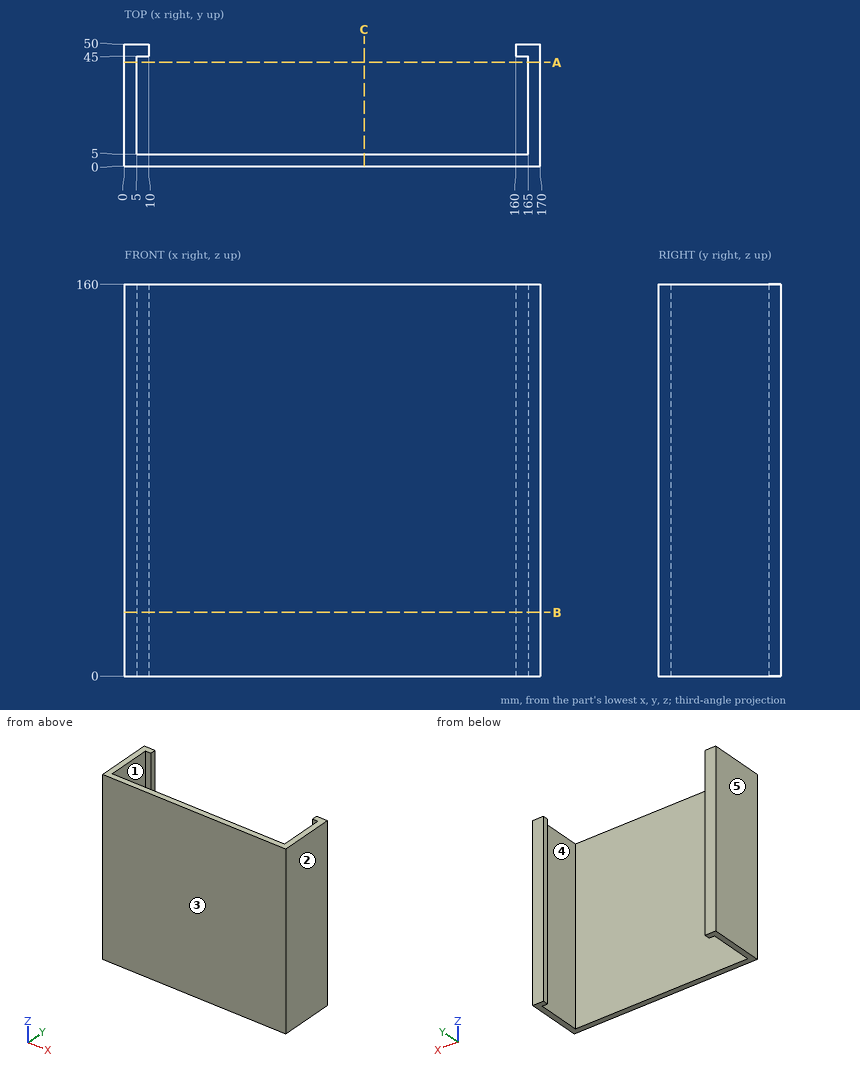
Geometry check sheet. Reference: drawing and pictorial views, mm from the part's lowest x, y, z. A direction names the side the tool comes from. Round coordinates to 2 decimals unless told otherwise and drop trailing zeros. Loops run counter-clockwise (first coordinate to the right, second up) from the corner with the lowest first, then second, coordinate; pieces in that order, holes last.
1. Scan lines: probe 1 along X at (y, z) = (47, 111.5); probe 2 along X at (y, z) = (38, 44.5); probe 3 along Y at (x, z) = (54, 127). Record each from-to range of solid material in increasing order.
2. Gauge pin test, flat end, axial feed: pin 1 Ø1.5 at (x, z) = (35, 46.5) entering from +Y. Record the tip position at first contact, or that the pin passes through.
3. Sectioned sample at A-A on y = 42.5. Record the boundary of the cut face in (x, z).
4. Sectioned sample at C-C on x = 98. Record the boundary of the cut face in (y, z).
5. Set-up check for the marked faces 4 and 5: record each of +Z, -Z, +X, -X, +Y, -Y from which the full face is reachable in a straight line by a thin tool's end or side.
6. Sectioned sample at B-B on z = 26. Record the boundary of the cut face in (x, y).
7. Mould release check, pull along Y, two halves, no side actions. Record for the marked faces 1, 2 and 3: released by +Y, released by -Y, zero draft, split by the parting line, or undercut.
Recorded:
1. probe 1: x = 0 to 10, 160 to 170
1. probe 2: x = 0 to 5, 165 to 170
1. probe 3: y = 0 to 5
2. pin 1: stops at y = 5
3. outline: (0, 0) - (5, 0) - (5, 160) - (0, 160) - close; (165, 0) - (170, 0) - (170, 160) - (165, 160) - close
4. outline: (0, 0) - (5, 0) - (5, 160) - (0, 160) - close
5. face 4: +Z, -Z
5. face 5: +Z, -Z, -X, +Y, -Y
6. outline: (0, 0) - (170, 0) - (170, 50) - (160, 50) - (160, 45) - (165, 45) - (165, 5) - (5, 5) - (5, 45) - (10, 45) - (10, 50) - (0, 50) - close
7. face 1: undercut
7. face 2: zero draft
7. face 3: released by -Y
